from build123d import *

# Parameters (mm, degrees)
SKETCH1_W                 = 56
SKETCH1_H                 = 106
BOSS_EXTRUDE1_DEPTH       = 5
SHELL1_T                  = -1.5
SHELL1_THICKNESS_2_FACE_W = 103
SHELL1_THICKNESS_2_FACE_H = 53
SHELL1_THICKNESS_2_DEPTH  = 1
SKETCH2_W                 = 36
SKETCH2_H                 = 48
CUT_EXTRUDE1_DEPTH        = 61.149812967
BOSS_EXTRUDE2_DEPTH       = 2.3
SKETCH4_R                 = 2.75
BOSS_EXTRUDE3_DEPTH       = 4.5
SKETCH5_R                 = 1.8
CUT_EXTRUDE2_DEPTH        = 4.5
MIRROR2_COPY_1_SKETCH_R   = 2.75
MIRROR2_COPY_1_DEPTH      = 4.5
MIRROR2_COPY_2_SKETCH_R   = 1.8
MIRROR2_COPY_2_DEPTH      = 4.5


with BuildPart() as part:
    # Sketch1 → Boss-Extrude1 (new body)
    with BuildSketch(Plane(origin=(0, 0, 0), x_dir=(1, 0, 0), z_dir=(0, 1, 0))):
        Rectangle(SKETCH1_W, SKETCH1_H)
    extrude(amount=-BOSS_EXTRUDE1_DEPTH)

    # Shell1
    shell1_openings = [part.faces().sort_by_distance(p)[0] for p in [
        (0, -5, 0),
    ]]
    offset(amount=SHELL1_T, openings=shell1_openings, kind=Kind.INTERSECTION)

    # Shell1 thickness 2 face (on inner face of the shell) → Shell1 thickness 2 (cut)
    with BuildSketch(Plane.ZX.offset(-1.5)):
        Rectangle(SHELL1_THICKNESS_2_FACE_W, SHELL1_THICKNESS_2_FACE_H)
    extrude(amount=SHELL1_THICKNESS_2_DEPTH, mode=Mode.SUBTRACT)

    # Sketch2 → Cut-Extrude1 (cut, through all)
    with BuildSketch(Plane(origin=(0, 0, 0), x_dir=(1, 0, 0), z_dir=(0, 1, 0))):
        with Locations((0, 24.4)):
            Rectangle(SKETCH2_W, SKETCH2_H)
    extrude(amount=-CUT_EXTRUDE1_DEPTH, mode=Mode.SUBTRACT)

    # Sketch3 → Boss-Extrude2 (add)
    with BuildSketch(Plane.XZ.offset(0.5)):
        Polygon((-21.6, -51.5), (21.6, -51.5), (21.6, 9.2), (18.1, 9.2), (18.1, 10.7), (23.1, 10.7), (23.1, -53), (-23.1, -53), (-23.1, 10.7), (-18.1, 10.7), (-18.1, 9.2), (-21.6, 9.2), align=None)
    extrude(amount=BOSS_EXTRUDE2_DEPTH)

    # Sketch4 → Boss-Extrude3 (add)
    with BuildSketch(Plane.XZ.offset(0.5)):
        with Locations((25.25, -50.25)):
            Circle(SKETCH4_R)
    boss_extrude3 = extrude(amount=BOSS_EXTRUDE3_DEPTH)

    # Sketch5 → Cut-Extrude2 (cut)
    with BuildSketch(Plane.XZ.offset(5)):
        with Locations(Location((25.25, -50.25, 0), (0, 0, 270))):
            Circle(SKETCH5_R)
    cut_extrude2 = extrude(amount=-CUT_EXTRUDE2_DEPTH, mode=Mode.SUBTRACT)

    # Mirror1: Boss-Extrude3, Cut-Extrude2 across plane
    add(boss_extrude3.mirror(Plane.XY))
    add(cut_extrude2.mirror(Plane.XY), mode=Mode.SUBTRACT)

    # Mirror2: Boss-Extrude3, Cut-Extrude2 across plane
    add(boss_extrude3.mirror(Plane(origin=(0, 0, 0), x_dir=(0, 0, 1), z_dir=(1, 0, 0))))
    add(cut_extrude2.mirror(Plane(origin=(0, 0, 0), x_dir=(0, 0, 1), z_dir=(1, 0, 0))), mode=Mode.SUBTRACT)

    # Mirror2 copy 1 sketch → Mirror2 copy 1 (add)
    with BuildSketch(Plane(origin=(0, -0.5, 0), x_dir=(-1, 0, 0), z_dir=(0, -1, 0))):
        with Locations((25.25, -50.25)):
            Circle(MIRROR2_COPY_1_SKETCH_R)
    extrude(amount=MIRROR2_COPY_1_DEPTH)

    # Mirror2 copy 2 sketch → Mirror2 copy 2 (cut)
    with BuildSketch(Plane(origin=(0, -5, 0), x_dir=(-1, 0, 0), z_dir=(0, -1, 0))):
        with Locations(Location((25.25, -50.25, 0), (0, 0, 270))):
            Circle(MIRROR2_COPY_2_SKETCH_R)
    extrude(amount=-MIRROR2_COPY_2_DEPTH, mode=Mode.SUBTRACT)


solid = part.part
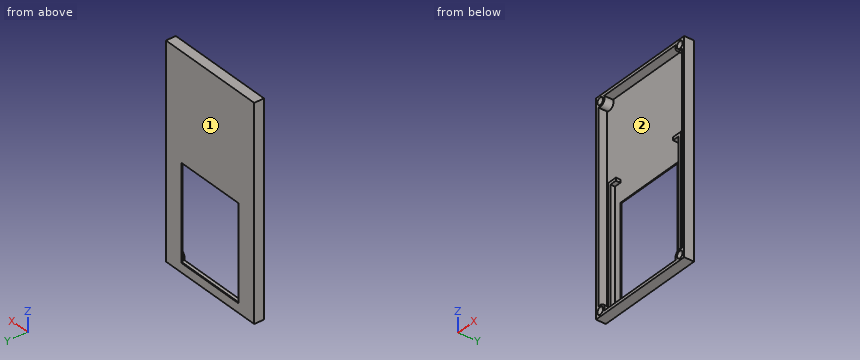
Model file for the job. Use its own axes, mm. Face numbers are marked on the shaded views. Give positions to 0.01 mm unless a question says otherwise; leave off trailing zeros. Order: outer loops, then holes, each group sorted by start corner. A loop starts at its lowest first (then second) coordinate and runs counter-clockwise, first axis right, second up. Notation, with made-up numbers: M 59.5,1 L 95.5,1 A15 cw 95.5,7 Z; hole C -40,-28.5 d3. An arc over 180 degrees is marked long. Put each result on its own line as item: value. Start each with the question number.
(1) Drill centre lines: L1, parallel to X at y = -2.7, z = 50.25; L2, parallel to X at y = -1.45, z = -50.25; L3, parallel to Z at x = -25.25, y = -3.3. Where is each one in solid material? Low to high. Write a range as [from, to].
(2) Pull direction X, two halves, no side cores. Call the marked faces 1 and 2: released by +X, released by -X, zero draft, split by the parting line, or undercut.
(3) Band-saw the part on D-D on x = -7.5. Give the cut face in (y, z), then the cut area to 3 significant figures.
(4) Pin check, flat tips, straight feed: pin 1 Ø3 at (x, z) = (25.25, -50.25) entering from -Y; pin 2 Ø4 at (x, z) = (20.5, -9.5) entering from -Y; pin 3 Ø3 at (x, z) = (25.5, -50.5) entering from -Y. Stop position of each tip, or through.
(5) Band-saw the part on B-B on z = -32. Give the cut face in (x, y), then the cut area to 3 significant figures.
(6) Band-saw the part on A-A on y = -1.9. Give the cut face in (x, z).
(7) Band-saw the part on C-C on x = 20.5. Give the cut face in (y, z).
Results below:
1. L1: x = [-28, -27.05], [-23.45, -22.5], [22.5, 23.45], [27.05, 28]
1. L2: x = [-28, -27.05], [-23.45, -21.6], [21.6, 23.45], [27.05, 28]
1. L3: z = [-53, -52.05], [-48.45, -47.5], [47.5, 48.45], [52.05, 53]
2. face 1: zero draft
2. face 2: undercut
3. outline: M -5,-53 L 0,-53 L 0,-48.4 L -0.5,-48.4 L -0.5,-51.5 L -5,-51.5 Z; M -5,51.5 L -0.5,51.5 L -0.5,-0.4 L 0,-0.4 L 0,53 L -5,53 Z
3. area: 42.5 mm2
4. pin 1: stops at y = -0.5
4. pin 2: stops at y = -2.8
4. pin 3: stops at y = -5
5. outline: M -28,-5 L -26.5,-5 L -26.5,-0.5 L -23.1,-0.5 L -23.1,-2.8 L -21.6,-2.8 L -21.6,-0.5 L -18,-0.5 L -18,0 L -28,0 Z; M 18,-0.5 L 21.6,-0.5 L 21.6,-2.8 L 23.1,-2.8 L 23.1,-0.5 L 26.5,-0.5 L 26.5,-5 L 28,-5 L 28,0 L 18,0 Z
5. area: 30.4 mm2
6. outline: M -28,-53 L 28,-53 L 28,53 L -28,53 Z; hole C -25.25,-50.25 d3.6; hole C -25.25,50.25 d3.6; hole M -26.5,-47.8 A2.75 cw -23.1,-48.54 L -23.1,10.7 L -18.1,10.7 L -18.1,9.2 L -21.6,9.2 L -21.6,-51.5 L 21.6,-51.5 L 21.6,9.2 L 18.1,9.2 L 18.1,10.7 L 23.1,10.7 L 23.1,-48.54 A2.75 cw 26.5,-47.8 L 26.5,47.8 A2.75 cw 22.8,51.5 L -22.8,51.5 A2.75 cw -26.5,47.8 Z; hole C 25.25,-50.25 d3.6; hole C 25.25,50.25 d3.6
7. outline: M -5,-53 L 0,-53 L 0,53 L -5,53 L -5,51.5 L -0.5,51.5 L -0.5,10.7 L -2.8,10.7 L -2.8,9.2 L -0.5,9.2 L -0.5,-51.5 L -5,-51.5 Z
